Input: part model. Units: mm. Frame: model coordinates. A direction names the side the tool comes from. Coordinates: 2 decimals unless noted, no trailing zeros. Loops run counter-clockwise (first coordinate to the right, second up) from the corner with the lowest first, then second, coordinate; pieces in that order, holes last.
(1) Mould query, pull axis Y, two halves, no side actions, for faces 1 (the face through (2.38, 10.74, 36.99)), 2 (the face through (-8, 8, 36)), 3 (the face through (12.85, 13.16, 6.12)). Classes: released by +Y, released by -Y, zero draft, split by the parting line, or undercut.
(2) Section A-A, the plane x = 0. Return loops of the section in (y, z).
(3) Section D-D, the plane y = -6. Return loops of the section in (x, z), then the cut area to 3 significant figures.
(4) Set-up query: faces 4 (the face through (-0.54, -2.44, 47.37)), 5 (the face through (-15.1, 15.1, 17.7)), 6 (the face through (-13.921, 12.155, 2.712)). Return all of +Z, -Z, +X, -X, +Y, -Y with unobstructed straight access to the full face (end or side cutting, diameter ignored); none if empty.
(5) Line query: L1, parallel to Y at x = 13, z = 3.5; L2, parallel to Z at x = -8.5, y = -10; L3, parallel to Z at x = 3, y = 7. Output: solid intervals per line, ascending.
(6) Section B-B, the plane y = 0. Return loops of the section in (x, z).
(7) Contact query for flat-ended pins moving along their axis: P1, Ø3, axis at x = 13, y = 13, coming from the +Z side; P2, Ø2, axis at x = 13, y = -13, coming from the -Z side; P3, Ø12, axis at y = 8, z = 43, coming from the -X side. Output: stop coordinate, or through.
(8) Section C-C, the plane z = 19.5. Return loops of the section in (x, y).
```python
from build123d import *

# Parameters (mm, degrees)
SKETCH1_W           = 35.2
SKETCH1_H           = 35.2
BOSS_EXTRUDE1_DEPTH = 36
SKETCH2_R           = 11
BOSS_EXTRUDE2_DEPTH = 2
SKETCH3_R           = 2.5
BOSS_EXTRUDE3_DEPTH = 19
CHAMFER1_SIZE       = 5
CIRPATTERN1_COUNT   = 4
SKETCH6_W           = 4.502968974
SKETCH6_H           = 1.338593798
CUT_EXTRUDE1_DEPTH  = 17


with BuildPart() as part:
    # Sketch1 → Boss-Extrude1 (new body)
    with BuildSketch(Plane.XY):
        Rectangle(SKETCH1_W, SKETCH1_H)
    extrude(amount=BOSS_EXTRUDE1_DEPTH)

    # Sketch2 → Boss-Extrude2 (add)
    with BuildSketch(Plane.XY.offset(36)):
        with Locations(Location((0, 0, 0), (0, 0, 180))):
            Circle(SKETCH2_R)
    extrude(amount=BOSS_EXTRUDE2_DEPTH)

    # Sketch3 → Boss-Extrude3 (add)
    with BuildSketch(Plane.XY.offset(38)):
        Circle(SKETCH3_R)
    extrude(amount=BOSS_EXTRUDE3_DEPTH)

    # Chamfer1
    chamfer1_edges = [part.edges().sort_by_distance(p)[0] for p in [
        (-17.6, 17.6, 18),
        (17.6, 17.6, 18),
        (17.6, -17.6, 18),
        (-17.6, -17.6, 18),
    ]]
    chamfer(chamfer1_edges, length=CHAMFER1_SIZE)

    # Sketch4 → M3x0.5 Tapped Hole1 (revolve, cut)
    with BuildSketch(Plane(origin=(13, 13, 36), x_dir=(0, -1, 0), z_dir=(1, 0, 0))):
        Polygon((0, 0), (0, 6.251075774), (1.25, 5.5), (1.25, 0), align=None)
    m3x0_5_tapped_hole1 = revolve(axis=Axis((13, 13, 42.35), (0, 0, -1)), mode=Mode.SUBTRACT)

    # CirPattern1: M3x0.5 Tapped Hole1 ×4 about axis
    cirpattern1_axis = Axis((0, 0, 0), (0, 0, 1))
    for i in range(1, CIRPATTERN1_COUNT):
        add(m3x0_5_tapped_hole1.rotate(cirpattern1_axis, i * 360 / CIRPATTERN1_COUNT), mode=Mode.SUBTRACT)

    # Sketch6 → Cut-Extrude1 (cut)
    with BuildSketch(Plane.XY.offset(57)):
        with Locations((-0.129996357, 2.669296899)):
            Rectangle(SKETCH6_W, SKETCH6_H)
    extrude(amount=-CUT_EXTRUDE1_DEPTH, mode=Mode.SUBTRACT)

    # Mirror1: M3x0.5 Tapped Hole1 across plane
    add(m3x0_5_tapped_hole1.mirror(Plane(origin=(0, 0, 18), x_dir=(1, 0, 0), z_dir=(0, 0, -1))), mode=Mode.SUBTRACT)

    # Mirror1 copy 1 sketch → Mirror1 copy 1 (revolve, cut)
    with BuildSketch(Plane(origin=(-13, 13, 0), x_dir=(1, 0, 0), z_dir=(0, 1, 0))):
        Polygon((0, 0), (0, -6.251075774), (1.25, -5.5), (1.25, 0), align=None)
    revolve(axis=Axis((-13, 13, -6.35), (0, 0, -1)), mode=Mode.SUBTRACT)

    # Mirror1 copy 2 sketch → Mirror1 copy 2 (revolve, cut)
    with BuildSketch(Plane(origin=(-13, -13, 0), x_dir=(0, 1, 0), z_dir=(-1, 0, 0))):
        Polygon((0, 0), (0, -6.251075774), (1.25, -5.5), (1.25, 0), align=None)
    revolve(axis=Axis((-13, -13, -6.35), (0, 0, -1)), mode=Mode.SUBTRACT)

    # Mirror1 copy 3 sketch → Mirror1 copy 3 (revolve, cut)
    with BuildSketch(Plane(origin=(13, -13, 0), x_dir=(-1, 0, 0), z_dir=(0, -1, 0))):
        Polygon((0, 0), (0, -6.251075774), (1.25, -5.5), (1.25, 0), align=None)
    revolve(axis=Axis((13, -13, -6.35), (0, 0, -1)), mode=Mode.SUBTRACT)


solid = part.part
```
Report:
1. face 1: split by the parting line
1. face 2: zero draft
1. face 3: undercut
2. outline: (-17.6, 0) - (17.6, 0) - (17.6, 36) - (11, 36) - (11, 38) - (2.5, 38) - (2.5, 40) - (2, 40) - (2, 57) - (-2.5, 57) - (-2.5, 38) - (-11, 38) - (-11, 36) - (-17.6, 36) - close
3. outline: (-17.6, 0) - (17.6, 0) - (17.6, 36) - (9.22, 36) - (9.22, 38) - (-9.22, 38) - (-9.22, 36) - (-17.6, 36) - close
3. area: 1,300 mm2
4. face 4: +Z
4. face 5: +Z, -Z, -X, +Y
4. face 6: -Z
5. L1: y = -17.2 to -14.25, -11.75 to 11.75, 14.25 to 17.2
5. L2: z = 0 to 36
5. L3: z = 0 to 38
6. outline: (-17.6, 0) - (17.6, 0) - (17.6, 36) - (11, 36) - (11, 38) - (2.5, 38) - (2.5, 57) - (-2.5, 57) - (-2.5, 38) - (-11, 38) - (-11, 36) - (-17.6, 36) - close
7. P1: stops at z = 36
7. P2: stops at z = 5.65
7. P3: stops at x = -9.95
8. outline: (-17.6, -12.6) - (-12.6, -17.6) - (12.6, -17.6) - (17.6, -12.6) - (17.6, 12.6) - (12.6, 17.6) - (-12.6, 17.6) - (-17.6, 12.6) - close
